```python
from build123d import *

# Parameters (mm, degrees)
BOSS_EXTRUDE1_DEPTH            = 42.8498
SKETCH4_R                      = 5.05
CUT_EXTRUDE1_DEPTH             = 1.524
F_1_16_0_0625_DIAMETER_HOLE1_D = 1.5875
F_1_8_0_125_DIAMETER_HOLE2_D   = 3.175


with BuildPart() as part:
    # Sketch1 → Boss-Extrude1 (new body)
    with BuildSketch(Plane.XY):
        with BuildLine():
            Line((-2.767900829, 5.715), (2.767900829, 5.715))
            ThreePointArc((2.767900829, 5.715), (4.490128061, 4.490128061), (5.715, 2.767900829))
            Line((5.715, 2.767900829), (5.715, -2.767900829))
            ThreePointArc((5.715, -2.767900829), (4.490128061, -4.490128061), (2.767900829, -5.715))
            Line((2.767900829, -5.715), (-2.767900829, -5.715))
            ThreePointArc((-2.767900829, -5.715), (-4.490128061, -4.490128061), (-5.715, -2.767900829))
            Line((-5.715, -2.767900829), (-5.715, 2.767900829))
            ThreePointArc((-5.715, 2.767900829), (-4.490128061, 4.490128061), (-2.767900829, 5.715))
        make_face()
    extrude(amount=BOSS_EXTRUDE1_DEPTH)

    # Sketch4 → Cut-Extrude1 (cut)
    with BuildSketch(Plane(origin=(0, 0, 0), x_dir=(-1, 0, 0), z_dir=(0, 0, -1))):
        Circle(SKETCH4_R)
    extrude(amount=-CUT_EXTRUDE1_DEPTH, mode=Mode.SUBTRACT)

    # 1/16 (0.0625) Diameter Hole1 (through all)
    with Locations(Plane(origin=(5.715, 0, 0), x_dir=(0, 0, -1), z_dir=(1, 0, 0))):
        with Locations((-1.524, 0)):
            Hole(F_1_16_0_0625_DIAMETER_HOLE1_D / 2)

    # 1/8 (0.125) Diameter Hole2 (through all)
    with Locations(Plane(origin=(0, 0, 1.524), x_dir=(-1, 0, 0), z_dir=(0, 0, -1))):
        with Locations((0, 0)):
            Hole(F_1_8_0_125_DIAMETER_HOLE2_D / 2)


solid = part.part
```
Design review of the part built by this model. Coordinates are the model's own, in mm. A direction names the side the tool comes from. Round coordinates to 2 decimals unless told otherwise and drop trailing zeros. Order: outer loops, then holes, each group sorted by start corner. A loop starts at its lowest first (then second) coordinate and runs counter-clockwise, first axis right, second up. Notation, with made-up numbers: (10.25, 20) - (66.25, 20) arc R10 ccw to (66.25, 28) - close; hole circle Ø3 at (-38.5, 82.25). An arc over 180 degrees is marked (long way). Return JSON: item names as keys, results as strings.
Q1. Wall thickness on L1, parallel to X at y = 0, z = 0.5 (3 decimals); L2, parallel to Z at x = 3.5, y = 3: over which ranges is each line inside the solid? List them lowest first. Write a range as [from, to].
Computed values:
{"L1": "x = [-5.715, -5.05], [5.05, 5.715]", "L2": "z = [1.52, 42.85]"}
Q2. Machinability: for faces 4 (the cylindrical face through (-4.06, 0.24, 2.28)), 5 (the flat face through (0, 2, 1.524)), which of the approach directions +Z, -Z, +X, -X, +Y, -Y give a long, thin tool a straight path to every point of the face, cutting with its end or side? Answer none if there is none.
Computed values:
{"face 4": "+X, -X", "face 5": "-Z"}
Q3. Consider section D-D on y = -4.25. Write out the cut boundary in (x, z).
Computed values:
{"outline": "(-4.72, 0) - (-2.73, 0) - (-2.73, 1.52) - (2.73, 1.52) - (2.73, 0) - (4.72, 0) - (4.72, 42.85) - (-4.72, 42.85) - close"}
Q4. For pin 1 Ø4.5 at (x, y) = (0, 2) entering from -Z; pin 2 Ø1.3 at (y, z) = (0, 1.524) entering from -X, all flat-tipped, find the tip position at first contact; note any pin that passes through.
Computed values:
{"pin 1": "stops at z = 1.52", "pin 2": "passes through"}
Q5. Consider section B-B on y = 0. Give the number of separate pieces and of enclosed holes in the cut face, plus the area to 3 significant figures.
Computed values:
{"separate pieces": "4", "enclosed holes": "0", "area": "336 mm2"}
Q6. The part is to be moulded in two halves that separate along X. For faces 1 (the cylindrical face through (4.51, -4.47, 21.12)), 2 (the cylindrical face through (-4.665, -1.934, 0.751)), 3 (the flat face through (0, 5.715, 21)), say which applies: pulls with the +X half, pulls with the -X half, needs draft (parallel to the pull), parting line crosses it, or undercut.
Computed values:
{"face 1": "pulls with the +X half", "face 2": "undercut", "face 3": "needs draft"}
